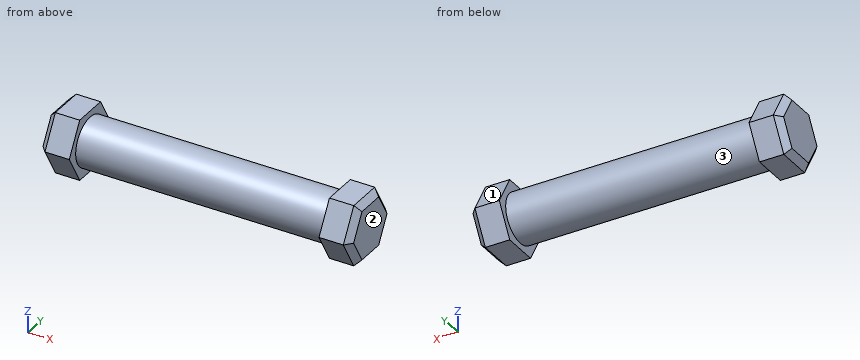
from build123d import *

# Parameters (mm, degrees)
F0_R     = 4
F1_DEPTH = 20.5
F3_DEPTH = 5
F4_SIZE  = 1


# Not quite as in the source:
# - a pattern or mirror of a feature is missing from the dataset's text; its kind, count and spacing are read off the source's solid


with BuildPart() as f1:
    # F0 (on Right) → F1 (new body, symmetric)
    with BuildSketch(Plane.YZ):
        Circle(F0_R)
    extrude(amount=F1_DEPTH, both=True)

    # F2 (on face) → F3 (join)
    with BuildSketch(Plane.YZ.offset(20.5)):
        Polygon((2.8867513459, 5), (-2.8867513459, 5), (-5.7735026919, 0), (-2.8867513459, -5), (2.8867513459, -5), (5.7735026919, 0), align=None)
    f3 = extrude(amount=F3_DEPTH)

    # F3_copies: F3 across plane
    add(f3.mirror(Plane(origin=(0, 0, 0), x_dir=(0, 0, -1), z_dir=(-1, 0, 0))))

    # F4
    f4_edges = [f1.edges().sort_by_distance(p)[0] for p in [
        (25.5, 4.330127, 2.5),
        (25.5, 0, 5),
        (25.5, -4.330127, 2.5),
        (25.5, -4.330127, -2.5),
        (25.5, 0, -5),
        (25.5, 4.330127, -2.5),
        (-25.5, 4.330127, 2.5),
        (-25.5, 4.330127, -2.5),
        (-25.5, 0, 5),
        (-25.5, -4.330127, 2.5),
        (-25.5, -4.330127, -2.5),
        (-25.5, 0, -5),
    ]]
    chamfer(f4_edges, length=F4_SIZE)


solid = f1.part
Work out the finished part from the listing and answer in its coordinate system (mm). Face numbers are marked on the shaded views. Give positions to 0.01 mm unless a question says otherwise; leave off trailing zeros. Write each loop counter-clockwise with the first axis right and the second up, starting at its lowest first coordinate (ties: lowest second). Pieces come first, ordered by that corner, then holes. Notation, with made-up numbers: (40.5, 21) - (84.5, 21) arc R32 ccw to (84.5, 58) - close; hole circle Ø6 at (-4, 56). An arc over 180 degrees is marked (long way). One line per item, written item: value. Start each with the question number.
1. Given pin 1 (6 mm diameter, centred on x = -11.5, y = 1.5, fed in from +Z); pin 2 (2 mm diameter, centred on x = 7.5, y = 4, fed in from +Z); pin 3 (2 mm diameter, centred on y = -4.5, z = 4, fed in from +X), each flat-ended and moving along its own axis, determine where each tip first touches the part or whether it passes through.
2. Consider probe 1 along X at (y, z) = (-4.25, -0.5); probe 2 along X at (y, z) = (-2.5, -4); probe 3 along Y at (x, z) = (-13.5, 1). Determine where each line is inside the solid, lowest interval first.
3. Find section C-C (x = 2). Write down the section's boundary in (y, z).
4. Find section B-B (y = 0). Write down the section's boundary in (x, z), then the cut area to 3 significant figures.
5. Find section A-A (z = -1.25). Write down the section's boundary in (x, y), then the cut area to 3 significant figures.
6. For a pull along X with two mould halves and no side action, classify the marked faces 1, 2 and 3 as +X half, -X half, draft (parallel to the pull), parting line (faces both ways), or undercut.
Geometry results:
1. pin 1: z = 4
1. pin 2: z = 2.65
1. pin 3: x = 24.6
2. probe 1: -25.5 to -20.5, 20.5 to 25.5
2. probe 2: -25.33 to -20.5, 20.5 to 25.33
2. probe 3: -3.87 to 3.87
3. outline: circle Ø8 at (0, 0)
4. outline: (-25.5, -4) - (-24.5, -5) - (-20.5, -5) - (-20.5, -4) - (20.5, -4) - (20.5, -5) - (24.5, -5) - (25.5, -4) - (25.5, 4) - (24.5, 5) - (20.5, 5) - (20.5, 4) - (-20.5, 4) - (-20.5, 5) - (-24.5, 5) - (-25.5, 4) - close
4. area: 426 mm2
5. outline: (-25.5, -3.9) - (-24.5, -5.05) - (-20.5, -5.05) - (-20.5, -3.8) - (20.5, -3.8) - (20.5, -5.05) - (24.5, -5.05) - (25.5, -3.9) - (25.5, 3.9) - (24.5, 5.05) - (20.5, 5.05) - (20.5, 3.8) - (-20.5, 3.8) - (-20.5, 5.05) - (-24.5, 5.05) - (-25.5, 3.9) - close
5. area: 410 mm2
6. face 1: draft
6. face 2: +X half
6. face 3: undercut
